The model under review builds one solid part; all positions refer to its coordinate system, in mm. Give positions to 0.01 mm unless a question says otherwise; leave off trailing zeros. Order: outer loops, then holes, each group sorted by start corner. A loop starts at its lowest first (then second) coordinate and runs counter-clockwise, first axis right, second up. Notation, with made-up numbers: (61, 62) -> (85, 62) arc R24 ccw to (85, 85) -> close; hole circle Ø11 at (60.5, 46.25). An arc over 180 degrees is marked (long way). Answer as a JSON object with one key per item and string values. Group by question number.
from build123d import *

# Parameters (mm, degrees)
EXTRUDE_1_DEPTH     = 20
SKETCH_2_R          = 2.1
CUT_EXTRUDE_2_DEPTH = 132.364611302
SKETCH_6_R          = 2.1
CUT_EXTRUDE_3_DEPTH = 117.990020748


with BuildPart() as part:
    # 草图1 → 凸台-拉伸1 (new body)
    with BuildSketch(Plane(origin=(0, 0, 0), x_dir=(1, 0, 0), z_dir=(0, 1, 0))):
        Polygon((90, 72.018504252), (-18.027756377, 0), (18.027756377, 0), (90, 47.981495748), align=None)
    extrude(amount=EXTRUDE_1_DEPTH)

    # 草图2 → 切除-拉伸2 (cut, through all)
    with BuildSketch(Plane(origin=(90, 0, 0), x_dir=(0, 0, -1), z_dir=(1, 0, 0))):
        with Locations((60, 10)):
            Circle(SKETCH_2_R)
    extrude(amount=-CUT_EXTRUDE_2_DEPTH, mode=Mode.SUBTRACT)

    # 草图6 → 切除-拉伸3 (cut, through all)
    with BuildSketch(Plane.XY):
        with Locations((0, 10)):
            Circle(SKETCH_6_R)
    extrude(amount=-CUT_EXTRUDE_3_DEPTH, mode=Mode.SUBTRACT)


solid = part.part
1. For pin 1 (8 mm diameter, centred on x = 26, y = 12, fed in from +Z); pin 2 (10 mm diameter, centred on x = 19, y = 13.5, fed in from -Z); pin 3 (8 mm diameter, centred on x = 58.5, y = 11.5, fed in from +Z); pin 4 (3.5 mm diameter, centred on y = 10, z = -60, fed in from +X), all flat-tipped, find the tip position at first contact; note any pin that passes through.
2. For probe 1 along Y at (x, z) = (80, -60); probe 2 along X at (y, z) = (10, -4.5); probe 3 along X at (y, z) = (10, -7), list the stretches that pass through material, from the lowest coordinate up. Write a range as [from, to].
3. Take a section at C-C on y = 10. Give the boundary of the cut face in (x, z), plus the area to 3 significant figures.
4. Take a section at B-B on z = -60. Give the boundary of the cut face in (x, y).
5. Take a section at D-D on y = 3.5. Give the boundary of the cut face in (x, z).
6. Take a section at A-A on x = 0. Give the boundary of the cut face in (y, z), plus the area to 3 significant figures.
7. Draft analysis for pull direction Z (two halves, no side actions). For faces 1 (the flat face through (90, 7.6, -59.8)), 2 (the cylindrical face through (81.86, 10.09, -57.9)), 3 (the flat face through (-0.3, 7.6, 0)), 4 (the flat face through (36.74, 9.86, -36.51)), state which applies: pulls with the +Z half, pulls with the -Z half, needs draft (parallel to the pull), parting line crosses it, or undercut.
Checks:
{
 "1": {"pin 1": "stops at z = -2.65", "pin 2": "stops at z = -28.02", "pin 3": "stops at z = -24.31", "pin 4": "passes through"},
 "2": {"probe 1": "y = [0, 7.9], [12.1, 20]", "probe 2": "x = [-11.28, -2.1], [2.1, 24.78]", "probe 3": "x = [-7.53, -2.1], [2.1, 28.53]"},
 "3": {"outline": "(-18.03, 0) -> (-2.1, -10.62) -> (-2.1, 0) -> close; (2.1, -13.42) -> (68.82, -57.9) -> (90, -57.9) -> (90, -47.98) -> (18.03, 0) -> (2.1, 0) -> close; (75.12, -62.1) -> (90, -72.02) -> (90, -62.1) -> close", "area": "2,040 mm2"},
 "4": {"outline": "(71.97, 0) -> (90, 0) -> (90, 7.9) -> (71.97, 7.9) -> close; (71.97, 12.1) -> (90, 12.1) -> (90, 20) -> (71.97, 20) -> close"},
 "5": {"outline": "(-18.03, 0) -> (90, -72.02) -> (90, -47.98) -> (18.03, 0) -> close"},
 "6": {"outline": "(0, -12.02) -> (7.9, -12.02) -> (7.9, 0) -> (0, 0) -> close; (12.1, -12.02) -> (20, -12.02) -> (20, 0) -> (12.1, 0) -> close", "area": "190 mm2"},
 "7": {"face 1": "needs draft", "face 2": "undercut", "face 3": "pulls with the +Z half", "face 4": "pulls with the -Z half"}
}
